Build history of the part. All positions in model axes, mm. Face numbers are marked on the shaded views. A direction names the side the tool comes from. Give positions to 0.01 mm unless a question says otherwise; leave off trailing zeros. Write each loop counter-clockwise with the first axis right and the second up, starting at its lowest first coordinate (ties: lowest second). Pieces come first, ordered by that corner, then holes. Notation, with made-up numbers: M 78.25,8 L 126.25,8 A32 ccw 126.25,35 Z; hole C -27.75,-8.75 d3. An arc over 180 degrees is marked long. Return JSON: item names as keys, results as strings. Group by question number.
Q1. Tool access for the marked faces 1, 2, 3, 4 and 5: list every direction of +Z, -Z, +X, -X, +Y, -Y with a clear straight run to the whole face (end or side of a thin tool).
Q2. Band-saw the part on A-A, the plane x = -37. Give the cut face in (y, z) (3 decimals), then the cut area to 3 significant figures.
Q3. Pull direction X, two halves, no side cores. Call the marked faces 6, 7 and 8: +X half, -X half, draft (parallel to the pull), parting line (faces both ways), or undercut.
Q4. Wall check: probe 1 along Z at (x, y) = (-30.5, 33); probe 2 along X at (y, z) = (32.5, 3); probe 3 along Z at (x, y) = (16, -3.5). Give the ranges that are in metal, low to high.
Q5. Band-saw the part on C-C, the plane x = 21.5. Give the cut face in (y, z) (3 decimals).
Q6. Flat gauge pins, fed straight in: pin 1 Ø3.5 at (y, z) = (17, 24.5) entering from -X; pin 2 Ø15.5 at (y, z) = (13.5, -54.5) entering from -X; pin 3 Ø9 at (y, z) = (20.5, -24.5) entering from +X; pin 4 Ø7.5 at (y, z) = (-12.192, 27.305) entering from +X. Where does each tip first touch, or does it go through?
Q7. Band-saw the part on D-D, the plane y = -2. Give the cut face in (x, z).
Q8. Band-saw the part on B-B, the plane z = -4. Give the cut face in (x, y), then the cut area to 3 significant figures.
from build123d import *

# Parameters (mm, degrees)
SKETCH1_W                = 88.9
SKETCH1_H                = 91.44
BOSS_EXTRUDE1_DEPTH      = 44.45
CUT_EXTRUDE1_DEPTH       = 38.1
CUT_EXTRUDE2_DEPTH       = 15.24
SKETCH4_R                = 6.64
CUT_EXTRUDE3_DEPTH       = 25.4
SKETCH5_W                = 13.209891204
SKETCH5_H                = 25.4
CUT_EXTRUDE4_DEPTH       = 12.7
BOSS_EXTRUDE2_DEPTH      = 25.4
BOSS_EXTRUDE2_DEPTH_BACK = 25.4
CUT_EXTRUDE6_DEPTH       = 45.72
CUT_EXTRUDE6_DEPTH_BACK  = 2.54
SKETCH9_W                = 12.7
SKETCH9_H                = 18.221589608
BOSS_EXTRUDE4_DEPTH      = 6.35
BOSS_EXTRUDE4_DEPTH_BACK = 6.35
BOSS_EXTRUDE6_DEPTH      = 38.1
SKETCH12_R               = 4.1
CUT_EXTRUDE7_DEPTH       = 98.736331214


with BuildPart() as part:
    # Sketch1 → Boss-Extrude1 (new body)
    with BuildSketch(Plane(origin=(0, 0, 0), x_dir=(1, 0, 0), z_dir=(0, 1, 0))):
        Rectangle(SKETCH1_W, SKETCH1_H)
    extrude(amount=BOSS_EXTRUDE1_DEPTH)

    # Sketch2 → Cut-Extrude1 (cut)
    with BuildSketch(Plane(origin=(0, 44.45, 0), x_dir=(1, 0, 0), z_dir=(0, 1, 0))):
        Polygon((-19.05, 30.48), (-19.05, -33.02), (3.496943095, -33.02), (3.496943095, -21.59), (18.736943095, -21.59), (18.736943095, -33.02), (31.75, -33.02), (31.75, 30.48), (18.736943095, 30.48), (18.736943095, 19.05), (3.496943095, 19.05), (3.496943095, 30.48), align=None)
    extrude(amount=-CUT_EXTRUDE1_DEPTH, mode=Mode.SUBTRACT)

    # Sketch3 → Cut-Extrude2 (cut)
    with BuildSketch(Plane.ZY.offset(-3.496943095)):
        with BuildLine():
            ThreePointArc((-24.765, 22.642), (-28.865, 18.542), (-24.765, 14.442))
            Line((-24.765, 14.442), (-24.765, 22.642))
        make_face()
        with BuildLine():
            Line((-24.765, 22.642), (-24.765, 14.442))
            ThreePointArc((-24.765, 14.442), (-21.865862197, 15.642862197), (-20.665, 18.542))
            ThreePointArc((-20.665, 18.542), (-21.865862197, 21.441137803), (-24.765, 22.642))
        make_face()
        with BuildLine():
            ThreePointArc((-24.765, 22.642), (-28.865, 18.542), (-24.765, 14.442))
            Line((-24.765, 14.442), (-24.765, 22.642))
        make_face()
        with BuildLine():
            Line((-24.765, 22.642), (-24.765, 14.442))
            ThreePointArc((-24.765, 14.442), (-21.865862197, 15.642862197), (-20.665, 18.542))
            ThreePointArc((-20.665, 18.542), (-21.865862197, 21.441137803), (-24.765, 22.642))
        make_face()
        with BuildLine():
            ThreePointArc((-24.765, 38.898), (-28.865, 34.798), (-24.765, 30.698))
            Line((-24.765, 30.698), (-24.765, 38.898))
        make_face()
        with BuildLine():
            Line((-24.765, 38.898), (-24.765, 30.698))
            ThreePointArc((-24.765, 30.698), (-21.865862197, 31.898862197), (-20.665, 34.798))
            ThreePointArc((-20.665, 34.798), (-21.865862197, 37.697137803), (-24.765, 38.898))
        make_face()
        with BuildLine():
            ThreePointArc((-24.765, 38.898), (-28.865, 34.798), (-24.765, 30.698))
            Line((-24.765, 30.698), (-24.765, 38.898))
        make_face()
        with BuildLine():
            Line((-24.765, 38.898), (-24.765, 30.698))
            ThreePointArc((-24.765, 30.698), (-21.865862197, 31.898862197), (-20.665, 34.798))
            ThreePointArc((-20.665, 34.798), (-21.865862197, 37.697137803), (-24.765, 38.898))
        make_face()
        with BuildLine():
            ThreePointArc((27.305, 22.642), (23.205, 18.542), (27.305, 14.442))
            Line((27.305, 14.442), (27.305, 22.642))
        make_face()
        with BuildLine():
            Line((27.305, 22.642), (27.305, 14.442))
            ThreePointArc((27.305, 14.442), (30.204137803, 15.642862197), (31.405, 18.542))
            ThreePointArc((31.405, 18.542), (30.204137803, 21.441137803), (27.305, 22.642))
        make_face()
        with BuildLine():
            ThreePointArc((27.305, 22.642), (23.205, 18.542), (27.305, 14.442))
            Line((27.305, 14.442), (27.305, 22.642))
        make_face()
        with BuildLine():
            Line((27.305, 22.642), (27.305, 14.442))
            ThreePointArc((27.305, 14.442), (30.204137803, 15.642862197), (31.405, 18.542))
            ThreePointArc((31.405, 18.542), (30.204137803, 21.441137803), (27.305, 22.642))
        make_face()
        with BuildLine():
            ThreePointArc((27.305, 38.898), (23.205, 34.798), (27.305, 30.698))
            Line((27.305, 30.698), (27.305, 38.898))
        make_face()
        with BuildLine():
            Line((27.305, 38.898), (27.305, 30.698))
            ThreePointArc((27.305, 30.698), (30.204137803, 31.898862197), (31.405, 34.798))
            ThreePointArc((31.405, 34.798), (30.204137803, 37.697137803), (27.305, 38.898))
        make_face()
        with BuildLine():
            ThreePointArc((27.305, 38.898), (23.205, 34.798), (27.305, 30.698))
            Line((27.305, 30.698), (27.305, 38.898))
        make_face()
        with BuildLine():
            Line((27.305, 38.898), (27.305, 30.698))
            ThreePointArc((27.305, 30.698), (30.204137803, 31.898862197), (31.405, 34.798))
            ThreePointArc((31.405, 34.798), (30.204137803, 37.697137803), (27.305, 38.898))
        make_face()
    extrude(amount=-CUT_EXTRUDE2_DEPTH, mode=Mode.SUBTRACT)

    # Sketch4 → Cut-Extrude3 (cut)
    with BuildSketch(Plane.ZY.offset(44.45)):
        with Locations((-24.765, 18.542)):
            Circle(SKETCH4_R)
        with Locations((-24.765, 34.798)):
            Circle(SKETCH4_R)
        with Locations((27.305, 18.542)):
            Circle(SKETCH4_R)
        with Locations((27.305, 34.798)):
            Circle(SKETCH4_R)
    extrude(amount=-CUT_EXTRUDE3_DEPTH, mode=Mode.SUBTRACT)

    # Sketch5 → Cut-Extrude4 (cut)
    with BuildSketch(Plane.ZY.offset(-31.75)):
        with Locations((-23.875054398, 25.4)):
            Rectangle(SKETCH5_W, SKETCH5_H)
    extrude(amount=-CUT_EXTRUDE4_DEPTH, mode=Mode.SUBTRACT)

    # Sketch8 → Boss-Extrude2 (add, two sides: drawn at the far end of the back side and taken through both)
    with BuildSketch(Plane(origin=(0, 0, 0), x_dir=(0, 0, -1), z_dir=(1, 0, 0)).offset(-BOSS_EXTRUDE2_DEPTH_BACK)):
        with BuildLine():
            ThreePointArc((48.846831284, 22.225), (52.699055938, 26.077224654), (56.551280591, 22.225))
            Line((56.551280591, 22.225), (59.678111875, 22.225))
            ThreePointArc((59.678111875, 22.225), (55.899195587, 35.347304601), (45.72, 44.45))
            Line((45.72, 44.45), (45.72, 22.225))
            Line((45.72, 22.225), (48.846831284, 22.225))
        make_face()
        with BuildLine():
            Line((59.678111875, 22.225), (56.551280591, 22.225))
            ThreePointArc((56.551280591, 22.225), (52.699055938, 18.372775346), (48.846831284, 22.225))
            Line((48.846831284, 22.225), (45.72, 22.225))
            Line((45.72, 22.225), (45.72, 0))
            ThreePointArc((45.72, 0), (55.899195587, 9.102695399), (59.678111875, 22.225))
        make_face()
        with BuildLine():
            ThreePointArc((48.846831284, 22.225), (52.699055938, 26.077224654), (56.551280591, 22.225))
            Line((56.551280591, 22.225), (59.678111875, 22.225))
            ThreePointArc((59.678111875, 22.225), (55.899195587, 35.347304601), (45.72, 44.45))
            Line((45.72, 44.45), (45.72, 22.225))
            Line((45.72, 22.225), (48.846831284, 22.225))
        make_face()
        with BuildLine():
            Line((59.678111875, 22.225), (56.551280591, 22.225))
            ThreePointArc((56.551280591, 22.225), (52.699055938, 18.372775346), (48.846831284, 22.225))
            Line((48.846831284, 22.225), (45.72, 22.225))
            Line((45.72, 22.225), (45.72, 0))
            ThreePointArc((45.72, 0), (55.899195587, 9.102695399), (59.678111875, 22.225))
        make_face()
    extrude(amount=BOSS_EXTRUDE2_DEPTH + BOSS_EXTRUDE2_DEPTH_BACK)

    # Sketch9 → Cut-Extrude6 (cut, two sides: drawn at the far end of the back side and taken through both)
    with BuildSketch(Plane(origin=(0, 0, 0), x_dir=(1, 0, 0), z_dir=(0, 1, 0)).offset(-CUT_EXTRUDE6_DEPTH_BACK)):
        with Locations((-6.35, 54.830794804)):
            Rectangle(SKETCH9_W, SKETCH9_H)
        with Locations((6.35, 54.830794804)):
            Rectangle(SKETCH9_W, SKETCH9_H)
    extrude(amount=CUT_EXTRUDE6_DEPTH + CUT_EXTRUDE6_DEPTH_BACK, mode=Mode.SUBTRACT)

    # Sketch10 → Boss-Extrude4 (add, two sides: drawn at the far end of the back side and taken through both)
    with BuildSketch(Plane(origin=(0, 0, 0), x_dir=(0, 0, -1), z_dir=(1, 0, 0)).offset(-BOSS_EXTRUDE4_DEPTH_BACK)):
        with BuildLine():
            Line((-45.72, 22.225), (-45.72, 44.45))
            ThreePointArc((-45.72, 44.45), (-56.029860076, 35.397643692), (-59.866502833, 22.225))
            Line((-59.866502833, 22.225), (-56.603251416, 22.225))
            ThreePointArc((-56.603251416, 22.225), (-52.793251416, 26.035), (-48.983251416, 22.225))
            Line((-48.983251416, 22.225), (-45.72, 22.225))
        make_face()
        with BuildLine():
            Line((-45.72, 0), (-45.72, 22.225))
            Line((-45.72, 22.225), (-48.983251416, 22.225))
            ThreePointArc((-48.983251416, 22.225), (-52.793251416, 18.415), (-56.603251416, 22.225))
            Line((-56.603251416, 22.225), (-59.866502833, 22.225))
            ThreePointArc((-59.866502833, 22.225), (-56.029860076, 9.052356308), (-45.72, 0))
        make_face()
        with BuildLine():
            Line((-45.72, 22.225), (-45.72, 44.45))
            ThreePointArc((-45.72, 44.45), (-56.029860076, 35.397643692), (-59.866502833, 22.225))
            Line((-59.866502833, 22.225), (-56.603251416, 22.225))
            ThreePointArc((-56.603251416, 22.225), (-52.793251416, 26.035), (-48.983251416, 22.225))
            Line((-48.983251416, 22.225), (-45.72, 22.225))
        make_face()
        with BuildLine():
            Line((-45.72, 0), (-45.72, 22.225))
            Line((-45.72, 22.225), (-48.983251416, 22.225))
            ThreePointArc((-48.983251416, 22.225), (-52.793251416, 18.415), (-56.603251416, 22.225))
            Line((-56.603251416, 22.225), (-59.866502833, 22.225))
            ThreePointArc((-59.866502833, 22.225), (-56.029860076, 9.052356308), (-45.72, 0))
        make_face()
    extrude(amount=BOSS_EXTRUDE4_DEPTH + BOSS_EXTRUDE4_DEPTH_BACK)

    # Sketch11 → Boss-Extrude6 (add)
    with BuildSketch(Plane.XZ):
        Polygon((18.736943095, 33.02), (18.736943095, 21.59), (3.496943095, 21.59), (3.496943095, 33.02), (3.496943095, 45.72), (18.736943095, 45.72), align=None)
        Polygon((18.736943095, -30.48), (18.736943095, -19.05), (3.496943095, -19.05), (3.496943095, -30.48), (3.496943095, -45.72), (18.736943095, -45.72), align=None)
    extrude(amount=BOSS_EXTRUDE6_DEPTH)

    # Sketch12 → Cut-Extrude7 (cut, through all)
    with BuildSketch(Plane(origin=(18.736943095, 0, 0), x_dir=(0, 0, -1), z_dir=(1, 0, 0))):
        with Locations((24.765, -12.192)):
            Circle(SKETCH12_R)
        with Locations((24.765, -28.448)):
            Circle(SKETCH12_R)
        with Locations((-27.305, -12.192)):
            Circle(SKETCH12_R)
        with Locations((-27.305, -28.448)):
            Circle(SKETCH12_R)
    extrude(amount=-CUT_EXTRUDE7_DEPTH, mode=Mode.SUBTRACT)


solid = part.part
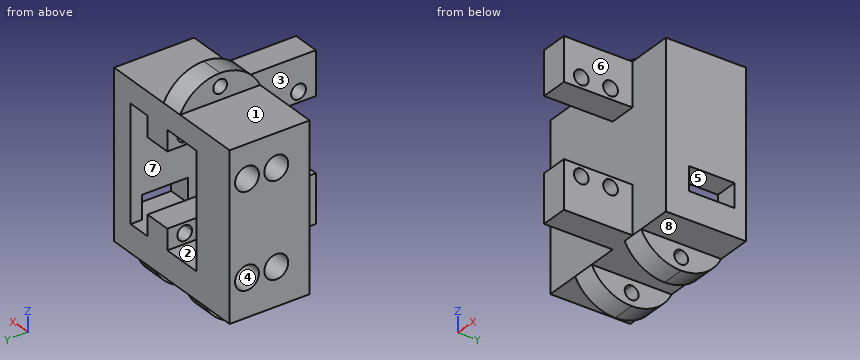
From the geometry:
{
 "1": {"face 1": "+Z, -X, +Y, -Y", "face 2": "+Y", "face 3": "+Z, -Z, -X, -Y", "face 4": "-X", "face 5": "+X"},
 "2": {"outline": "M 0,-45.72 L 44.45,-45.72 L 44.45,45.72 L 0,45.72 Z; hole C 18.542,-24.765 d13.28; hole C 18.542,27.305 d13.28; hole C 34.798,-24.765 d13.28; hole C 34.798,27.305 d13.28", "area": "3,510 mm^2"},
 "3": {"face 6": "+X half", "face 7": "undercut", "face 8": "draft"},
 "4": {"probe 1": "z = -45.72 to -31.16, -18.37 to 20.91, 33.7 to 45.72", "probe 2": "x = -44.45 to -19.05, 31.75 to 44.45", "probe 3": "z = -45.72 to -19.05, 21.59 to 45.72"},
 "5": {"outline": "M 0,-45.72 A24.673 ccw 44.45,-45.72 L 44.45,-30.48 L 6.35,-30.48 L 6.35,33.02 L 44.45,33.02 L 44.45,45.72 L 0,45.72 Z; hole C 22.225,-52.699 d7.704"},
 "6": {"pin 1": "stops at x = 3.5", "pin 2": "stops at x = -25.4", "pin 3": "stops at x = 18.74", "pin 4": "passes through"},
 "7": {"outline": "M 3.5,-45.72 L 18.74,-45.72 L 18.74,-19.05 L 3.5,-19.05 Z; M 3.5,21.59 L 18.74,21.59 L 18.74,45.72 L 3.5,45.72 Z"},
 "8": {"outline": "M -44.45,0 L 44.45,0 L 44.45,44.45 L 31.75,44.45 L 31.75,6.35 L -19.05,6.35 L -19.05,44.45 L -44.45,44.45 Z", "area": "2,020 mm^2"}
}
